CAD build for the part. Positions are in the model's coordinates, mm. Face numbers are marked on the shaded views. Give positions to 0.01 mm unless a question says otherwise; leave off trailing zeros. Write each loop counter-clockwise with the first axis right and the second up, starting at its lowest first coordinate (ties: lowest second). Pieces come first, ordered by that corner, then holes. Notation, with made-up numbers: M 43.25,16.25 L 49.25,16.25 A26 ccw 49.25,37.25 Z; hole C 63.5,-8 d9. An arc over 180 degrees is marked long. One line per question, with ' | ' between items. Start each with the question number.
1. Wall check: L1, parallel to Y at x = -4.75, z = 1.45; L2, parallel to Y at x = -4.25, z = 0.95; L3, parallel to X at y = 6.5, z = 0.3. Give the ranges that are in metal, low to high.
2. Pull direction X, two halves, no side cores. Call the marked faces 1, 2, 3 and 4: released by +X, released by -X, zero draft, split by the parting line, or undercut.
3. Cut at B-B, the plane x = -4.95. Write the cut outline in (y, z).
4. Cut at A-A, the plane y = 5. Write the cut outline in (x, z), then the cut area to 3 significant figures.
5. Cut at C-C, the plane z = 2.9. Write the cut outline in (x, y).
6. Flat gauge pin, fed straight in: pin 1 (4.5 mm diameter, centred on x = -4.95, y = 5, fed in from +Z). Where does the tip first touch, or does it go through?
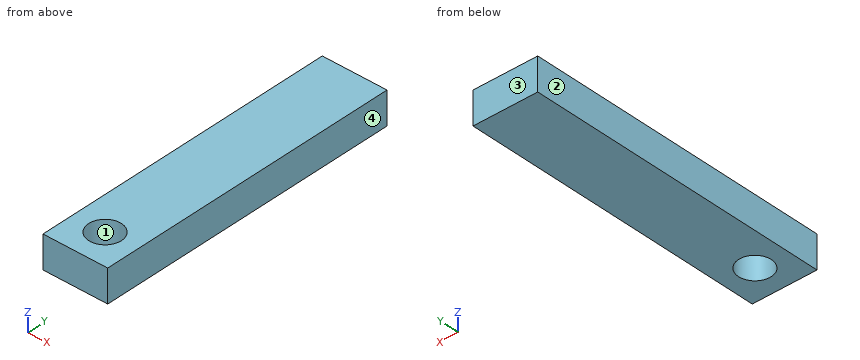
Autodesk Inventor part; units mm, degrees
ref_plane "YZ Plane" through (0, 0, 0) normal (1, 0, 0) x (0, 1, 0)
ref_plane "XZ Plane" through (0, 0, 0) normal (0, 1, 0) x (-1, 0, 0)
ref_plane "XY Plane" through (0, 0, 0) normal (0, 0, 1) x (1, 0, 0)
sketch "Sketch2" plane through (0, 0, 0) normal (0, 0, 1) x (1, 0, 0)
  line L0 (0, 0) -> (-9.9, 0)
  line L1 (-9.9, 0) -> (-9.9, 105)
  line L2 (-9.9, 105) -> (0, 105)
  line L3 (0, 105) -> (0, 0)
  line L4 (-4.95, 0) -> (-4.95, 2.5)
  line L5 (-4.95, 0) -> (-2.45, 0) construction
  circle A0 centre (-4.95, 5) radius 2.5
  line L6 (-4.95, 7.5) -> (32.05, 7.5) construction
  line L7 (0, 44.5) -> (0, 0)
  line L8 (0, 0) -> (-9.9, 0)
  line L9 (-9.9, 0) -> (-9.9, 44.5)
  line L10 (0, 45.5) -> (0, 0)
  line L11 (0, 0) -> (-9.9, 0)
  line L12 (-9.9, 0) -> (-9.9, 45.5)
  line L13 (-4.95, 7.5) -> (66.05, 7.5) construction
  line L14 (-9.9, 78.5) -> (0, 78.5)
  line L15 (0, 0) -> (-9.9, 0)
  line L16 (-9.9, 0) -> (-9.9, 47)
  line L17 (-9.9, 47) -> (0, 47)
  line L18 (0, 47) -> (0, 0)
  dimension "d35" = 5
  dimension "d4" = 9.9
  dimension "d5" = 105
  dimension "d33" = 2.5
  dimension "d34" = 90
  dimension "d46" = 9.9
  dimension "d47" = 47
extrude "Extrusion6" add sketch "Sketch2" along normal blind 5 contours L0 L1 L17 L3
properties part number "Elbow_Cube_Holder_TestFit_V2"
Here are the results:
1) L1: 0 to 2.51, 7.49 to 47 | L2: 0 to 2.6, 7.4 to 47 | L3: -9.9 to -6.95, -2.95 to 0
2) face 1: undercut | face 2: released by -X | face 3: zero draft | face 4: released by +X
3) outline: M 0,0 L 2.5,0 L 2.5,5 L 0,5 Z; M 7.5,0 L 47,0 L 47,5 L 7.5,5 Z
4) outline: M -9.9,0 L -7.45,0 L -7.45,5 L -9.9,5 Z; M -2.45,0 L 0,0 L 0,5 L -2.45,5 Z | area: 24.5 mm^2
5) outline: M -9.9,0 L 0,0 L 0,47 L -9.9,47 Z; hole C -4.95,5 d5
6) pin 1: through
